Source: CAD feature listing. Evaluate the final solid. Frame: model axes, mm. Coordinates: 2 decimals unless noted, no trailing zeros. One line per item, written item: value. Start each with the question number.
1. First-contact query: P1, Ø3, axis at x = 30, y = 58.5, coming from the -Z side. Flat tip, straight axial feed; report the tip coordinate or a pass-through.
2. Section query A-A, the plane z = 3. State how many separate pieces and enclosed holes the cut face has, and give its area (3 significant figures).
3. Line query: line 1 (X direction, y = 114.3, z = 4.5); line 2 (X direction, y = 42.5, z = 2.75); line 3 (X direction, y = 116.5, z = 6) (3 decimals). Output: solid intervals per line, ascending.
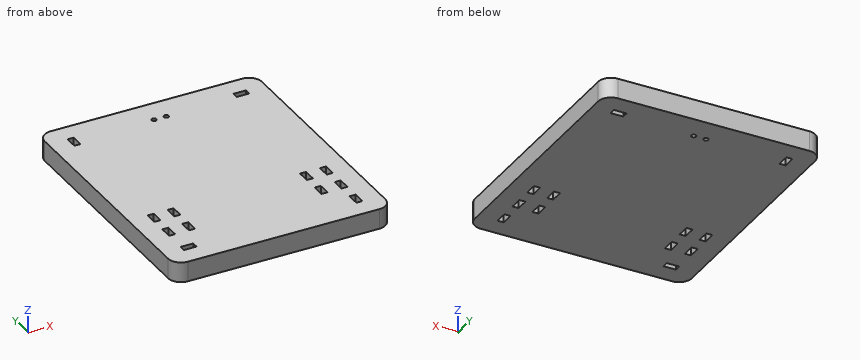
from build123d import *

# Parameters (mm, degrees)
SKETCH1_R           = 1.1938
SKETCH1_W           = 6.2611
SKETCH1_H           = 3.04
SKETCH1_W_2         = 3.04
SKETCH1_H_2         = 6.2611
SKETCH1_H_3         = 6.2541
BOSS_EXTRUDE1_DEPTH = 10


with BuildPart() as part:
    # Sketch1 → Boss-Extrude1 (new body)
    with BuildSketch(Plane.XY):
        with BuildLine():
            Line((-0.021357312, 120.65), (-0.021357312, 6.35000179))
            ThreePointArc((-0.021357312, 6.35000179), (1.838514627, 1.85987373), (6.328642688, 1.79e-06))
            Line((6.328642688, 1.79e-06), (101.6, 1.79e-06))
            ThreePointArc((101.6, 1.79e-06), (106.090128061, 1.85987373), (107.95, 6.35000179))
            Line((107.95, 6.35000179), (107.95, 120.65))
            ThreePointArc((107.95, 120.65), (106.090128061, 125.140128061), (101.6, 127))
            Line((101.6, 127), (6.328642688, 127))
            ThreePointArc((6.328642688, 127), (1.838514627, 125.140128061), (-0.021357312, 120.65))
        make_face()
        with Locations((50.927, 114.3)):
            Circle(SKETCH1_R, mode=Mode.SUBTRACT)
        with Locations((57.023, 114.3)):
            Circle(SKETCH1_R, mode=Mode.SUBTRACT)
        with Locations((12.723092688, 11.1339)):
            Rectangle(SKETCH1_W, SKETCH1_H, mode=Mode.SUBTRACT)
        with Locations((95.20555, 115.86610179)):
            Rectangle(SKETCH1_W, SKETCH1_H, mode=Mode.SUBTRACT)
        with Locations((11.112542688, 114.25555179)):
            Rectangle(SKETCH1_W_2, SKETCH1_H_2, mode=Mode.SUBTRACT)
        with Locations((11.112542688, 26.59548464)):
            Rectangle(SKETCH1_W_2, SKETCH1_H_3, mode=Mode.SUBTRACT)
        with Locations((96.8161, 26.59548464)):
            Rectangle(SKETCH1_W_2, SKETCH1_H_3, mode=Mode.SUBTRACT)
        with Locations((11.112542688, 40.17738464)):
            Rectangle(SKETCH1_W_2, SKETCH1_H_3, mode=Mode.SUBTRACT)
        with Locations((96.8161, 12.74445)):
            Rectangle(SKETCH1_W_2, SKETCH1_H_2, mode=Mode.SUBTRACT)
        with Locations((96.8161, 40.17738464)):
            Rectangle(SKETCH1_W_2, SKETCH1_H_3, mode=Mode.SUBTRACT)
        with Locations((21.010542688, 26.59548464)):
            Rectangle(SKETCH1_W_2, SKETCH1_H_3, mode=Mode.SUBTRACT)
        with Locations((21.010542688, 40.17738464)):
            Rectangle(SKETCH1_W_2, SKETCH1_H_3, mode=Mode.SUBTRACT)
        with Locations((86.9181, 26.59548464)):
            Rectangle(SKETCH1_W_2, SKETCH1_H_3, mode=Mode.SUBTRACT)
        with Locations((86.9181, 40.17738464)):
            Rectangle(SKETCH1_W_2, SKETCH1_H_3, mode=Mode.SUBTRACT)
    extrude(amount=BOSS_EXTRUDE1_DEPTH)


solid = part.part
Computed values:
1. P1: stops at z = 0
2. separate pieces: 1
2. enclosed holes: 14
2. area: 13,400 mm²
3. line 1: x = -0.02 to 9.59, 12.63 to 49.73, 52.12 to 55.83, 58.22 to 107.95
3. line 2: x = -0.02 to 9.59, 12.63 to 19.49, 22.53 to 85.4, 88.44 to 95.3, 98.34 to 107.95
3. line 3: x = -0.021 to 9.593, 12.633 to 92.075, 98.336 to 107.95
